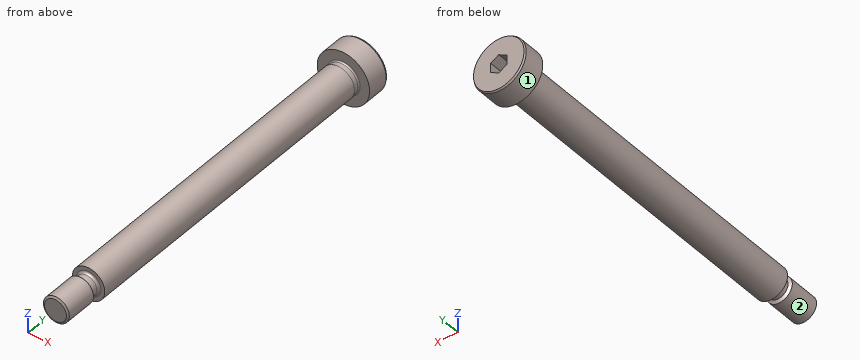
Autodesk Inventor part; units mm, degrees
ref_plane "YZ Plane" through (0, 0, 0) normal (1, 0, 0) x (0, 1, 0)
ref_plane "XZ Plane" through (0, 0, 0) normal (0, 1, 0) x (-1, 0, 0)
ref_plane "XY Plane" through (0, 0, 0) normal (0, 0, 1) x (1, 0, 0)
sketch "Sketch1" plane through (0, 0, 0) normal (0, 0, 1) x (1, 0, 0)
  line L0 (-2.5718, -2.6632) -> (-7.5718, -2.6632)
  line L1 (-7.5718, -2.6632) -> (-7.5718, -100.8132)
  line L2 (-7.5718, -100.8132) -> (-2.5718, -100.8132)
  line L3 (-2.5718, -100.8132) -> (-2.5718, -2.6632)
  dimension "d1" = 98.15
  dimension "d2" = 5
revolve "Shoulder" add sketch "Sketch1" angle 360 about axis through (-2.5718, -100.8132, 0) along (0, 1, 0)
sketch "Sketch2" plane through (-2.5718, -2.6632, 0) normal (0, 1, 0) x (1, 0, 0)
  circle A0 centre (0, 0) radius 5
  circle A1 centre (0, 0) radius 4.76
  dimension "d3" = 9.52
extrude "Shoulder_neck" add sketch "Sketch2" along normal blind 1.85 contours A1
sketch "Sketch3" plane through (-2.5718, -0.8132, 0) normal (0, 1, 0) x (1, 0, 0)
  circle A0 centre (0, 0) radius 4.76
  circle A1 centre (0, 0) radius 8.1
  dimension "d6" = 16.2
extrude "Head" add sketch "Sketch3" along normal blind 7 contours A0 | A1
sketch "Sketch4" plane through (-2.5718, -100.8132, 0) normal (0, -1, 0) x (1, 0, 0)
  circle A0 centre (0, 0) radius 5
  circle A1 centre (0, 0) radius 3.09
  dimension "d9" = 6.18
extrude "Thread_neck" add sketch "Sketch4" along normal blind 2.6 contours A1
sketch "Sketch5" plane through (-2.5718, -103.4132, 0) normal (0, -1, 0) x (1, 0, 0)
  circle A0 centre (0, 0) radius 3.09
  circle A1 centre (0, 0) radius 4
  dimension "d12" = 8
extrude "Thread_shoulder" add sketch "Sketch5" along normal blind 10.4 contours A0 | A1
sketch "Sketch6" plane through (-2.5718, 6.1868, 0) normal (0, 1, 0) x (1, 0, 0)
  circle A0 centre (0, 0) radius 8.1
  circle A1 centre (0, 0) radius 2.5 construction
  line L0 (-2.5, 1.4434) -> (-2.5, -1.4434)
  line L1 (-2.5, -1.4434) -> (0, -2.8868)
  line L2 (0, -2.8868) -> (2.5, -1.4434)
  line L3 (2.5, -1.4434) -> (2.5, 1.4434)
  line L4 (2.5, 1.4434) -> (0, 2.8868)
  line L5 (0, 2.8868) -> (-2.5, 1.4434)
  dimension "d15" = 5
extrude "Hex" cut sketch "Sketch6" against normal blind 4.2 contours L5 L4 L3 L2 L1 L0
chamfer "Chamfer1" distance 0.24 angle 30 1 edges at (2.4282, -2.6632, 0) measured on face at (-7.3973, -2.6632, -0.7786)
fillet "Fillet1" radius 0.4 1 edges at (-7.3318, -0.8132, 0)
chamfer "Chamfer2" distance 0.5 angle 30 1 edges at (-10.6718, 6.1868, 0) measured on face at (5.4233, 3.8535, 1.2993)
chamfer "Chamfer3" distance 0.625 angle 30 1 edges at (-6.5718, -113.8132, 0) measured on face at (-1.8144, -113.8132, 1.0973)
fillet "Fillet2" radius 0.7 1 edges at (-5.6618, -100.8132, 0)
chamfer "Chamfer7" distance 0.91 angle 30 1 edges at (-6.5718, -103.4132, 0) measured on face at (1.0861, -103.4132, -0.3191)
thread "Thread"
equation "\"d1\" = Shoulder_length - Shoulder_neck_length"
equation "\"d2\" = 0.5 * Shoulder_diameter"
equation "\"d3\" = Shoulder_neck_dia"
equation "\"d4\" = Shoulder_neck_length"
equation "\"d6\" = Head_diameter"
equation "\"d7\" = Head_height"
equation "\"d9\" = Thread_neck_dia"
equation "\"d10\" = Thread_neck_length"
equation "\"d12\" = Thread_diameter"
equation "\"d13\" = Thread_length - Thread_neck_length"
equation "\"d15\" = Hex_size"
equation "\"d16\" = Hex_length"
equation "\"d18\" = -0.5 * Shoulder_neck_dia + 0.5 * Shoulder_diameter"
equation "\"d64\" = -0.5 * Shoulder_neck_dia + 0.5 * Shoulder_diameter"
equation "\"d21\" = 0.1 * Hex_size"
equation "\"d65\" = 0.1 * Hex_size"
equation "\"d23\" = 0.5 * Thread_pitch"
equation "\"d66\" = 0.5 * Thread_pitch"
equation "\"d25\" = Thread_neck_radius"
equation "\"d60\" = -0.5 * Thread_neck_dia + 0.5 * Thread_diameter"
equation "\"d67\" = -0.5 * Thread_neck_dia + 0.5 * Thread_diameter"
equation "\"Shoulder_length\" = 100"
equation "\"Shoulder_neck_dia\" = 9.52"
equation "\"Thread_diameter\" = 8"
equation "\"Thread_length\" = 13"
equation "\"Head_diameter\" = 16.2"
equation "\"Head_height\" = 7"
equation "\"Thread_neck_dia\" = 6.18"
equation "\"Hex_size\" = 5"
equation "\"Hex_length\" = 4.2"
equation "\"Thread_pitch\" = 1.25"
equation "\"Shoulder_neck_length\" = 1.85"
equation "\"Thread_neck_length\" = 2.6"
equation "\"Thread_neck_radius\" = 0.7"
properties part number "SCREW, SHOULDER, P, 12.9,  M10X100MM" material "Steel, High Strength Low Alloy"
Could you check a few things on this model? Use its own coordinates, in mm. Face numbers are marked on the shaded views. A direction names the side the tool comes from. Give positions to 0.01 mm unless a question says otherwise; leave off trailing zeros. Write each loop counter-clockwise with the first axis right and the second up, starting at its lowest first coordinate (ties: lowest second). Pieces come first, ordered by that corner, then holes. Notation, with made-up numbers: (19, -28) -> (29, -28) arc R31 ccw to (29, 1) -> close; hole circle Ø8 at (-14.5, 18.5). An arc over 180 degrees is marked (long way). Answer as CSV lines item,"result". Start each with the question number.
(1) Which directions (+Z, -Z, +X, -X, +Y, -Y) give clear straight access to the entire face, cutting with the end or side of a thin tool? Please do the marked faces 1 and 2.
(2) I'm going to push flat-ended pins straight in: pin 1 Ø1 at (x, y) = (-3.5, -94.5) entering from +Z; pin 2 Ø1.5 at (x, y) = (-1, -25) entering from -Z; pin 3 Ø2.5 at (x, z) = (-3.5, 0.5) entering from +Y. Where does each tip first touch, or does it pass through?
(3) If we section it at A-A, the plane y = -21: Write out the boundary of the cut face in (x, z), and give its area (3 significant figures).
(4) Please list where these lines run through material, in increasing order: line 1 (Y direction, x = -1.5, z = 6.5); line 2 (X direction, y = -69, z = 3); line 3 (Z direction, x = -2.5, y = -48.5).
Answer list:
1,face 1,"+Y, -Y"
1,face 2,"-Y"
2,pin 1,"z = 4.98"
2,pin 2,"z = -4.93"
2,pin 3,"y = 1.99"
3,outline,"circle Ø10 at (-2.57, 0)"
3,area,"78.5 mm^2"
4,line 1,"-0.81 to 6.19"
4,line 2,"-6.57 to 1.43"
4,line 3,"-5 to 5"
